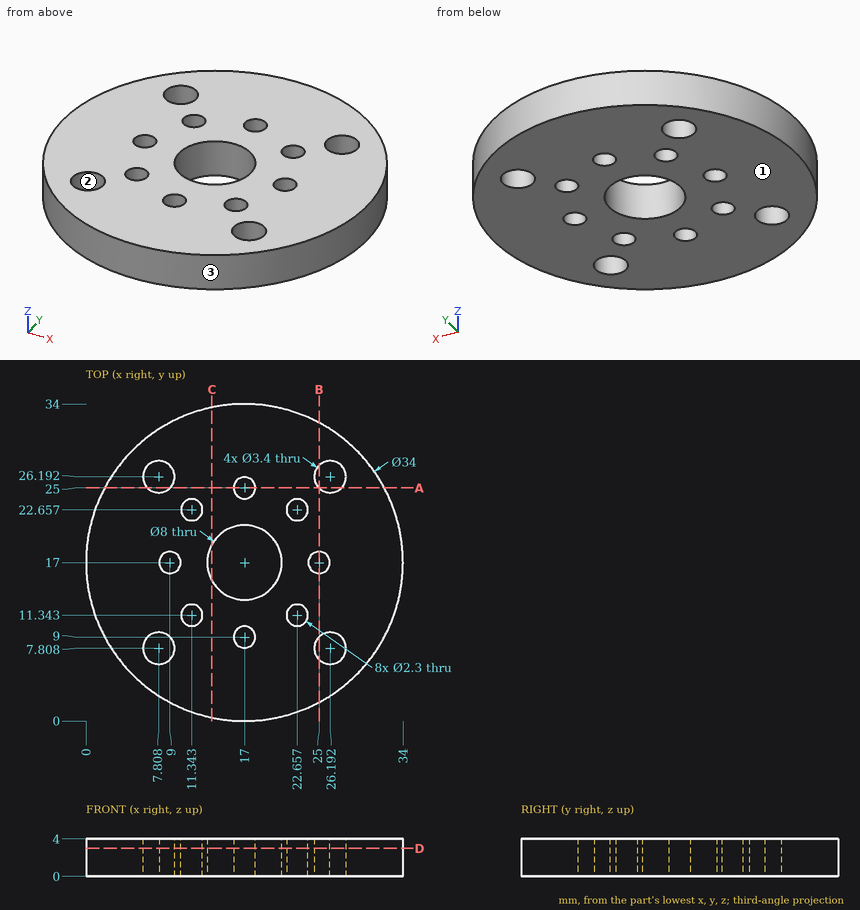
The drawing under review shows one solid part. Ordinate dimensions are in mm from its lowest x, y, z. Coordinates: 2 decimals unless noted, no trailing zeros. Write each loop counter-clockwise with the first axis right and the second up, starting at its lowest first coordinate (ties: lowest second). Pieces come first, ordered by that corner, then holes.
1) Add section D-D (z = 3). State how many separate pieces and enclosed holes the cut face has, plus the area to 3 significant figures.
2) Add section C-C (x = 13.5). Write out the cut boundary in (y, z) (1 decimal).
3) To check wall thickness, follow L1, parallel to Y at x = 17, z = 2.1; L2, parallel to X at y = 12, z = 1.85; L3, parallel to X at y = 8, z = 3.2 (1 decimal). State the ranges of each line that lie inside material, in increasing order.
4) Add section A-A (y = 25). Write out the cut boundary in (x, z).
5) Insertion check: pin 1 (2 mm diameter, centred on x = 9, y = 17, fed in from -Z); pin 2 (1.5 mm diameter, centred on x = 12.5, z = 2, fed in from -Y). Each pin has a flat end and moves straight along its axis. Give the tip position at first contact, or say it passes through.
6) Mouldability with a two-part tool opening along X and no side actions: class the marked faces 1, 2 and 3 as +X half, -X half, draft (parallel to the pull), parting line (faces both ways), or undercut.
Check result:
1. separate pieces: 1
1. enclosed holes: 13
1. area: 788 mm2
2. outline: (0.4, 0) - (15.1, 0) - (15.1, 4) - (0.4, 4) - close; (18.9, 0) - (33.6, 0) - (33.6, 4) - (18.9, 4) - close
3. L1: y = 0 to 7.85, 10.15 to 13, 21 to 23.85, 26.15 to 34
3. L2: x = 0.75 to 10.4, 12.29 to 21.71, 23.6 to 33.25
3. L3: x = 2.6 to 6.1, 9.5 to 16.4, 17.6 to 24.5, 27.9 to 31.4
4. outline: (2, 0) - (6.6, 0) - (6.6, 4) - (2, 4) - close; (9.02, 0) - (15.85, 0) - (15.85, 4) - (9.02, 4) - close; (18.15, 0) - (24.98, 0) - (24.98, 4) - (18.15, 4) - close; (27.4, 0) - (32, 0) - (32, 4) - (27.4, 4) - close
5. pin 1: passes through
5. pin 2: stops at y = 0.42
6. face 1: draft
6. face 2: undercut
6. face 3: parting line
